```python
from build123d import *

# Parameters (mm, degrees)
SKETCH_1_R          = 5
SKETCH_1_R_2        = 9.5
SKETCH_1_R_3        = 1.5
EXTRUDE_1_DEPTH     = 8
SKETCH_2_R          = 11
CUT_EXTRUDE_1_DEPTH = 2


with BuildPart() as part:
    # Эскиз1 → Бобышка-Вытянуть1 (new body)
    with BuildSketch(Plane.XY):
        with BuildLine():
            Line((32, -50), (32, -17))
            Line((32, -17), (32, 12))
            ThreePointArc((32, 12), (31.121320344, 14.121320344), (29, 15))
            Line((29, 15), (-29, 15))
            ThreePointArc((-29, 15), (-31.121320344, 14.121320344), (-32, 12))
            Line((-32, 12), (-32, -17))
            Line((-32, -17), (-32, -30.127300246))
            ThreePointArc((-32, -30.127300246), (-32.109032978, -30.77864019), (-32.424243723, -31.358962601))
            Line((-32.424243723, -31.358962601), (-41.119742613, -42.483754153))
            ThreePointArc((-41.119742613, -42.483754153), (-41.434953358, -43.064076563), (-41.543986336, -43.715416508))
            Line((-41.543986336, -43.715416508), (-41.543986336, -52.683803611))
            Line((-41.543986336, -52.683803611), (-41.543986336, -53.383022016))
            ThreePointArc((-41.543986336, -53.383022016), (-40.958199899, -54.797235578), (-39.543986336, -55.383022016))
            Line((-39.543986336, -55.383022016), (-32.37679771, -55.383022016))
            ThreePointArc((-32.37679771, -55.383022016), (-31.741748464, -55.610550363), (-31.395682628, -56.189597106))
            ThreePointArc((-31.395682628, -56.189597106), (3.109514103, -81.848562323), (32, -50))
        make_face()
        Circle(SKETCH_1_R, mode=Mode.SUBTRACT)
        with Locations((-19, 0)):
            Circle(SKETCH_1_R_2, mode=Mode.SUBTRACT)
        with Locations((19, 0)):
            Circle(SKETCH_1_R_2, mode=Mode.SUBTRACT)
        with Locations((-5.656854249, 5.656854249)):
            Circle(SKETCH_1_R_3, mode=Mode.SUBTRACT)
        with Locations((5.656854249, 5.656854249)):
            Circle(SKETCH_1_R_3, mode=Mode.SUBTRACT)
        with Locations((5.656854249, -5.656854249)):
            Circle(SKETCH_1_R_3, mode=Mode.SUBTRACT)
        with Locations((-5.656854249, -5.656854249)):
            Circle(SKETCH_1_R_3, mode=Mode.SUBTRACT)
        with Locations((-9.5, 12)):
            Circle(SKETCH_1_R_3, mode=Mode.SUBTRACT)
        with Locations((9.5, 12)):
            Circle(SKETCH_1_R_3, mode=Mode.SUBTRACT)
        with Locations((9.5, -12)):
            Circle(SKETCH_1_R_3, mode=Mode.SUBTRACT)
        with Locations((-9.5, -12)):
            Circle(SKETCH_1_R_3, mode=Mode.SUBTRACT)
        with Locations((-25.902777778, -31.358962601)):
            Circle(SKETCH_1_R_3, mode=Mode.SUBTRACT)
        with Locations((26, -31.358962601)):
            Circle(SKETCH_1_R_3, mode=Mode.SUBTRACT)
        with BuildLine():
            ThreePointArc((-25.902777778, -52.246353355), (26, -50), (-25.902777778, -47.753646645))
            ThreePointArc((-25.902777778, -47.753646645), (-26.099772408, -48.268225789), (-26.539423077, -48.600349063))
            ThreePointArc((-26.539423077, -48.600349063), (-27.5, -50), (-26.539423077, -51.399650937))
            ThreePointArc((-26.539423077, -51.399650937), (-26.099772408, -51.731774211), (-25.902777778, -52.246353355))
        make_face(mode=Mode.SUBTRACT)
    extrude(amount=EXTRUDE_1_DEPTH)

    # Эскиз2 → Вырез-Вытянуть1 (cut)
    with BuildSketch(Plane.XY.offset(8)):
        Circle(SKETCH_2_R)
    extrude(amount=-CUT_EXTRUDE_1_DEPTH, mode=Mode.SUBTRACT)


solid = part.part
```
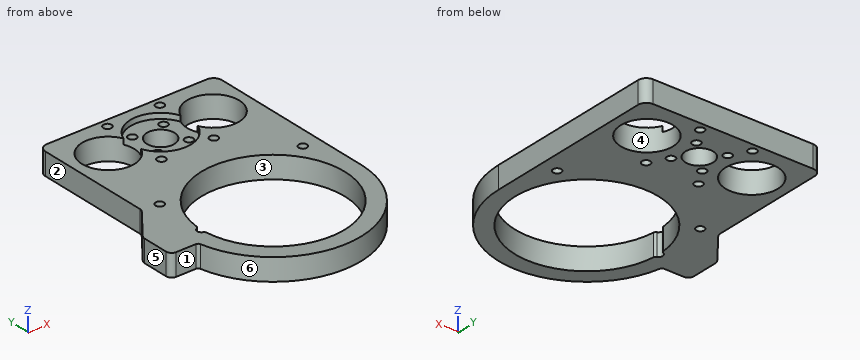
The listing builds one solid part. Answer for the finished solid, in the listing's coordinates (mm). Face numbers are marked on the shaded views. A direction names the side the tool comes from. Give positions to 0.01 mm unless a question says otherwise; leave off trailing zeros. Order: outer loops, then holes, each group sorted by start corner. A loop starts at its lowest first (then second) coordinate and runs counter-clockwise, first axis right, second up.
1) Consider line 1 along Y through (x, z) = (0, 3.8); line 2 along Y through (x, z) = (-20.5, 3.5); line 3 along X through (y, z) = (2, 2.25). Determine where each line is inside the solid, lowest interval first.
Reported:
line 1: y = -82 to -76, -24 to -5, 5 to 15
line 2: y = -74.57 to -65.99, -34.01 to -9.38, 9.38 to 15
line 3: x = -32 to -28.29, -9.71 to -4.58, 4.58 to 9.71, 28.29 to 32
2) For the marked faces 1, 2 and 3, determine the directions among +Z, -Z, +X, -X, +Y, -Y from which every point of the face is accessible in a straight line to the end or side of a thin tool.
Reported:
face 1: +Z, -Z, -X, -Y
face 2: +Z, -Z, -X, +Y
face 3: +Z, -Z
3) Find section C-C on z = 3.25. Give the number of separate pieces and of enclosed holes in the cut face, then the cut area to 3 significant figures.
Reported:
separate pieces: 1
enclosed holes: 14
area: 3,100 mm2
4) Find section D-D on x = 19. Write down the section's boundary in (y, z), then the cut area to 3 significant figures.
Reported:
outline: (-75.75, 0) - (-67.75, 0) - (-67.75, 8) - (-75.75, 8) - close; (-32.25, 0) - (-9.5, 0) - (-9.5, 8) - (-32.25, 8) - close; (9.5, 0) - (15, 0) - (15, 8) - (9.5, 8) - close
area: 290 mm2
5) Given P1, Ø4, axis at y = -3.5, z = 3.5, coming from the -X side; P2, Ø3.5, axis at x = -5.66, y = 5.66, coming from the +Z side; P3, Ø4, axis at y = -67.5, z = 6, coming from the -X side, each flat-ended and moving along its own axis, determine where each tip first touches the part or whether it passes through.
Reported:
P1: stops at x = -32
P2: stops at z = 6
P3: stops at x = -28
6) Find section A-A on y = 0. Write down the section's boundary in (x, z).
Reported:
outline: (-32, 0) - (-28.5, 0) - (-28.5, 8) - (-32, 8) - close; (-9.5, 0) - (-5, 0) - (-5, 6) - (-9.5, 6) - close; (5, 0) - (9.5, 0) - (9.5, 6) - (5, 6) - close; (28.5, 0) - (32, 0) - (32, 8) - (28.5, 8) - close
7) Determine the mould class of the marked faces 4, 5 and 6 for opening direction Y: pulls with the +Y half, pulls with the -Y half, needs draft (parallel to the pull), parting line crosses it, or undercut.
Reported:
face 4: undercut
face 5: needs draft
face 6: pulls with the -Y half
8) Find section B-B on x = 0. Write down the section's boundary in (y, z).
Reported:
outline: (-82, 0) - (-76, 0) - (-76, 8) - (-82, 8) - close; (-24, 0) - (-5, 0) - (-5, 6) - (-11, 6) - (-11, 8) - (-24, 8) - close; (5, 0) - (15, 0) - (15, 8) - (11, 8) - (11, 6) - (5, 6) - close
